Build history of the part. All positions in model axes, mm. Round coordinates to 2 decimals unless told otherwise and drop trailing zeros. Write each loop counter-clockwise with the first axis right and the second up, starting at its lowest first coordinate (ties: lowest second). Pieces come first, ordered by that corner, then holes. Notation, with made-up numbers: (-25.75, 81) - (-6.75, 81) arc R24 cw to (-6.75, 116) - close; hole circle Ø7 at (-24, 63.25). An arc over 180 degrees is marked (long way). Answer as a JSON object with one key per item and string values. Group by question number.
Item 1: Slice it at D-D, the plane z = 1.5. Give the number of separate pieces and of enclosed holes in the cut face, then the cut area to 3 significant figures.
Item 2: Probe line 1 (X direction, y = -33, z = 2.45); line 2 (X direction, y = 6, z = 0.25); line 3 (Y direction, x = -38.5, z = 0.7). List the from-to ranges inside material, lowest first. Write a range as from..to.
Item 3: Slice it at B-B, the plane y = -5. List the corners of the cut face in (x, z), then the cut area to 3 significant figures.
Item 4: Slice it at A-A, the plane x = 20.5. List the corners of the cut face in (y, z), then the cut area to 3 significant figures.
Item 5: Slice it at C-C, the plane y = -31. List the corners of the cut face in (x, z), then the cut area to 3 significant figures.
from build123d import *

# Parameters (mm, degrees)
F0_R     = 4.75
F1_DEPTH = 3


with BuildPart() as f1:
    # F0 (on Top) → F1 (new body)
    with BuildSketch(Plane.XY):
        with BuildLine():
            ThreePointArc((0, 11), (-7.778175, -7.778175), (11, 0))
            ThreePointArc((11, 0), (7.778175, 7.778175), (0, 11))
        make_face()
        with BuildLine():
            ThreePointArc((4.75, 41), (-3.358757, 44.358757), (0, 36.25))
            ThreePointArc((0, 36.25), (3.358757, 37.641243), (4.75, 41))
        make_face()
        with BuildLine():
            ThreePointArc((-4.358899, 32), (-9.997173, 23.23776), (-4.781818, 14.217391))
            ThreePointArc((-4.781818, 14.217391), (-8.816779, 12.135255), (-12.04388, 8.941195))
            ThreePointArc((-12.04388, 8.941195), (-19.011127, 16.688739), (-29.086835, 14.034103))
            ThreePointArc((-29.086835, 14.034103), (-48.503882, 15.759867), (-31.780782, 5.742985))
            ThreePointArc((-31.780782, 5.742985), (-25.18972, -2.327014), (-14.999206, -0.154364))
            ThreePointArc((-14.999206, -0.154364), (-14.265848, -4.635255), (-12.225345, -8.691429))
            ThreePointArc((-12.225345, -8.691429), (-21.746696, -12.923552), (-22.335551, -23.326447))
            ThreePointArc((-22.335551, -23.326447), (-29.977048, -41.259867), (-15.282705, -28.45064))
            ThreePointArc((-15.282705, -28.45064), (-5.57093, -24.675934), (-4.488201, -14.312793))
            ThreePointArc((-4.488201, -14.312793), (0, -15), (4.488201, -14.312793))
            ThreePointArc((4.488201, -14.312793), (5.57093, -24.675934), (15.282705, -28.45064))
            ThreePointArc((15.282705, -28.45064), (29.977048, -41.259867), (22.335551, -23.326447))
            ThreePointArc((22.335551, -23.326447), (21.746696, -12.923552), (12.225345, -8.691429))
            ThreePointArc((12.225345, -8.691429), (14.265848, -4.635255), (14.999206, -0.154364))
            ThreePointArc((14.999206, -0.154364), (25.18972, -2.327014), (31.780782, 5.742985))
            ThreePointArc((31.780782, 5.742985), (48.503882, 15.759867), (29.086835, 14.034103))
            ThreePointArc((29.086835, 14.034103), (19.011127, 16.688739), (12.04388, 8.941195))
            ThreePointArc((12.04388, 8.941195), (8.816779, 12.135255), (4.781818, 14.217391))
            ThreePointArc((4.781818, 14.217391), (9.997173, 23.23776), (4.358899, 32))
            ThreePointArc((4.358899, 32), (0, 51), (-4.358899, 32))
        make_face()
        with BuildLine():
            ThreePointArc((-26.891175, -37.012527), (-26.25565, -28.937416), (-19.349195, -33.169697))
            ThreePointArc((-19.349195, -33.169697), (-21.94274, -37.401978), (-26.891175, -37.012527))
        make_face(mode=Mode.SUBTRACT)
        with Locations((-13.519061, -18.607391)):
            Circle(F0_R, mode=Mode.SUBTRACT)
        with BuildLine():
            ThreePointArc((0, 11), (7.778175, 7.778175), (11, 0))
            ThreePointArc((11, 0), (-7.778175, -7.778175), (0, 11))
        make_face(mode=Mode.SUBTRACT)
        with Locations((24.099195, -33.169697)):
            Circle(F0_R, mode=Mode.SUBTRACT)
        with Locations((13.519061, -18.607391)):
            Circle(F0_R, mode=Mode.SUBTRACT)
        with Locations((-38.993317, 12.669697)):
            Circle(F0_R, mode=Mode.SUBTRACT)
        with Locations((-21.8743, 7.107391)):
            Circle(F0_R, mode=Mode.SUBTRACT)
        with BuildLine():
            ThreePointArc((4.75, 23), (3.358757, 19.641243), (0, 18.25))
            ThreePointArc((0, 18.25), (-4.75, 23), (0, 27.75))
            ThreePointArc((0, 27.75), (3.358757, 26.358757), (4.75, 23))
        make_face(mode=Mode.SUBTRACT)
        with BuildLine():
            ThreePointArc((4.75, 41), (3.358757, 37.641243), (0, 36.25))
            ThreePointArc((0, 36.25), (-3.358757, 44.358757), (4.75, 41))
        make_face(mode=Mode.SUBTRACT)
        with Locations((21.8743, 7.107391)):
            Circle(F0_R, mode=Mode.SUBTRACT)
        with Locations((38.993317, 12.669697)):
            Circle(F0_R, mode=Mode.SUBTRACT)
    extrude(amount=F1_DEPTH)


solid = f1.part
Geometry says:
{
 "1": {"separate pieces": "1", "enclosed holes": "11", "area": "2,640 mm^2"},
 "2": {"line 1": "x = -34.1..-28.85, -19.35..-14.1, 14.1..19.35, 28.85..34.1", "line 2": "x = -46.44..-26.49, -17.26..-9.22, 9.22..17.26, 26.49..46.44", "line 3": "y = 2.68..7.95, 17.39..22.66"},
 "3": {"outline": "(-14.14, 0) - (-9.8, 0) - (-9.8, 3) - (-14.14, 3) - close; (9.8, 0) - (14.14, 0) - (14.14, 3) - (9.8, 3) - close", "area": "26.1 mm^2"},
 "4": {"outline": "(-42.5, 0) - (-36.27, 0) - (-36.27, 3) - (-42.5, 3) - close; (-30.07, 0) - (-11.45, 0) - (-11.45, 3) - (-30.07, 3) - close; (-2.8, 0) - (2.56, 0) - (2.56, 3) - (-2.8, 3) - close; (11.65, 0) - (17.01, 0) - (17.01, 3) - (11.65, 3) - close", "area": "107 mm^2"},
 "5": {"outline": "(-33.86, 0) - (-28.32, 0) - (-28.32, 3) - (-33.86, 3) - close; (-19.87, 0) - (-14.34, 0) - (-14.34, 3) - (-19.87, 3) - close; (14.34, 0) - (19.87, 0) - (19.87, 3) - (14.34, 3) - close; (28.32, 0) - (33.86, 0) - (33.86, 3) - (28.32, 3) - close", "area": "66.4 mm^2"}
}
